Part model, mm, in its own coordinate system. Give positions to 0.01 mm unless a question says otherwise; leave off trailing zeros. Order: outer loops, then holes, each group sorted by start corner. A loop starts at its lowest first (then second) coordinate and runs counter-clockwise, first axis right, second up. Notation, with made-up numbers: M -2,-27 L 45,-27 A22 cw 45,-4 Z; hole C -35,-31 d5. An arc over 180 degrees is marked long. One line per question, with ' | ' between items.
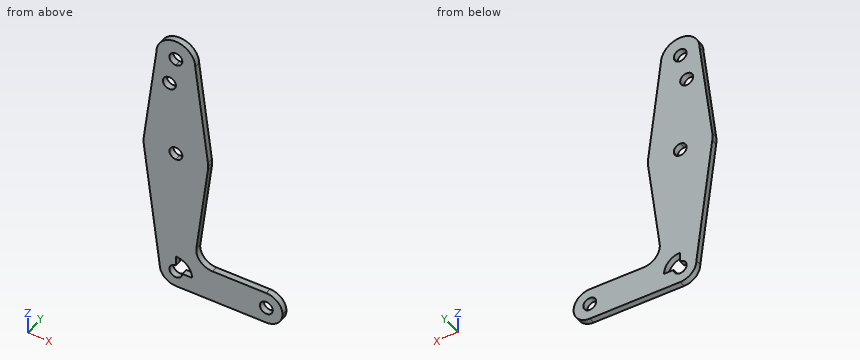
```python
from build123d import *

# Parameters (mm, degrees)
F0_R     = 3.175
F1_DEPTH = 3.048


with BuildPart() as f1:
    # F0 (on Front) → F1 (new body)
    with BuildSketch(Plane.XZ):
        with BuildLine():
            ThreePointArc((3.175, 0), (-2.2450640303, -2.2450640303), (0, 3.175))
            Line((0, 3.175), (0, 7.9375))
            ThreePointArc((0, 7.9375), (-5.6126600757, 5.6126600757), (-7.9375, 0))
            ThreePointArc((-7.9375, 0), (-5.6126600757, -5.6126600757), (0, -7.9375))
            ThreePointArc((0, -7.9375), (5.6126600757, -5.6126600757), (7.9375, 0))
            Line((7.9375, 0), (3.175, 0))
        make_face()
        with BuildLine():
            ThreePointArc((-7.9375, 0), (-5.6126600757, 5.6126600757), (0, 7.9375))
            Line((0, 7.9375), (0, 47.625))
            ThreePointArc((0, 47.625), (-10.4943466753, 51.5884798259), (-15.7484878283, 61.4998109785))
            Line((-15.7484878283, 61.4998109785), (-7.9375, 0))
        make_face()
        with BuildLine():
            Line((0, 47.625), (0, 7.9375))
            ThreePointArc((0, 7.9375), (5.6126600757, 5.6126600757), (7.9375, 0))
            Line((7.9375, 0), (36.5125, 0))
            ThreePointArc((36.5125, 0), (38.8373399243, 5.6126600757), (44.45, 7.9375))
            Line((44.45, 7.9375), (17.969436389, 7.9375))
            ThreePointArc((17.969436389, 7.9375), (12.0041470858, 10.632131185), (10.0825936846, 16.8893946619))
            Line((10.0825936846, 16.8893946619), (15.7484878283, 61.4998109785))
            ThreePointArc((15.7484878283, 61.4998109785), (10.4943466753, 51.5884798259), (0, 47.625))
        make_face()
        with BuildLine():
            Line((36.5125, 0), (7.9375, 0))
            ThreePointArc((7.9375, 0), (5.6126600757, -5.6126600757), (0, -7.9375))
            Line((0, -7.9375), (44.45, -7.9375))
            ThreePointArc((44.45, -7.9375), (38.8373399243, -5.6126600757), (36.5125, 0))
        make_face()
        with BuildLine():
            ThreePointArc((-15.7484878283, 61.4998109785), (-10.4943466753, 51.5884798259), (0, 47.625))
            Line((0, 47.625), (0, 60.325))
            ThreePointArc((0, 60.325), (-3.175, 63.5), (0, 66.675))
            Line((0, 66.675), (0, 79.375))
            ThreePointArc((0, 79.375), (-10.4912828548, 75.4142187767), (-15.7474569047, 65.5082893304))
            ThreePointArc((-15.7474569047, 65.5082893304), (-15.874999475, 63.504082824), (-15.7484878283, 61.4998109785))
        make_face()
        with BuildLine():
            Line((0, 60.325), (0, 47.625))
            ThreePointArc((0, 47.625), (10.4943466753, 51.5884798259), (15.7484878283, 61.4998109785))
            ThreePointArc((15.7484878283, 61.4998109785), (15.8433403876, 62.4979070089), (15.875, 63.5))
            ThreePointArc((15.875, 63.5), (15.8430821396, 64.5061676396), (15.7474569047, 65.5082893304))
            ThreePointArc((15.7474569047, 65.5082893304), (10.4912828548, 75.4142187767), (0, 79.375))
            Line((0, 79.375), (0, 66.675))
            ThreePointArc((0, 66.675), (2.2450640303, 65.7450640303), (3.175, 63.5))
            ThreePointArc((3.175, 63.5), (2.2450640303, 61.2549359697), (0, 60.325))
        make_face()
        with BuildLine():
            ThreePointArc((44.45, 7.9375), (38.8373399243, 5.6126600757), (36.5125, 0))
            ThreePointArc((36.5125, 0), (38.8373399243, -5.6126600757), (44.45, -7.9375))
            ThreePointArc((44.45, -7.9375), (50.0626600757, -5.6126600757), (52.3875, 0))
            ThreePointArc((52.3875, 0), (50.0626600757, 5.6126600757), (44.45, 7.9375))
        make_face()
        with BuildLine():
            ThreePointArc((47.625, 0), (44.45, -3.175), (41.275, 0))
            ThreePointArc((41.275, 0), (44.45, 3.175), (47.625, 0))
        make_face(mode=Mode.SUBTRACT)
        with BuildLine():
            Line((-9.525, 114.3), (-15.7474569047, 65.5082893304))
            ThreePointArc((-15.7474569047, 65.5082893304), (-10.4912828548, 75.4142187767), (0, 79.375))
            Line((0, 79.375), (0, 100.0252))
            Line((0, 100.0252), (0, 104.775))
            ThreePointArc((0, 104.775), (-6.7351920908, 107.5648079092), (-9.525, 114.3))
        make_face()
        with Locations((-3.175, 100.0252)):
            Circle(F0_R, mode=Mode.SUBTRACT)
        with BuildLine():
            Line((0, 100.0252), (0, 79.375))
            ThreePointArc((0, 79.375), (10.4912828548, 75.4142187767), (15.7474569047, 65.5082893304))
            Line((15.7474569047, 65.5082893304), (9.525, 114.3))
            ThreePointArc((9.525, 114.3), (6.7351920908, 107.5648079092), (0, 104.775))
            Line((0, 104.775), (0, 100.0252))
        make_face()
        with BuildLine():
            ThreePointArc((9.525, 114.3), (0, 123.825), (-9.525, 114.3))
            ThreePointArc((-9.525, 114.3), (-6.7351920908, 107.5648079092), (0, 104.775))
            ThreePointArc((0, 104.775), (6.7351920908, 107.5648079092), (9.525, 114.3))
        make_face()
        with BuildLine():
            ThreePointArc((3.175, 114.3), (2.2450640303, 112.0549359697), (0, 111.125))
            ThreePointArc((0, 111.125), (-2.2450640303, 116.5450640303), (3.175, 114.3))
        make_face(mode=Mode.SUBTRACT)
    extrude(amount=F1_DEPTH)


solid = f1.part
```
1. Slice it at B-B on y = -1.1. Give the number of separate pieces and of enclosed holes in the cut face, then the cut area to 3 significant figures.
Worked out:
separate pieces: 1 | enclosed holes: 5 | area: 3,560 mm2
2. Drop flat-ended pins along their axis: pin 1 (1.5 mm diameter, centred on x = 5, y = -1, fed in from +Z); pin 2 (1.5 mm diameter, centred on y = -1.5, z = 6, fed in from +X); pin 3 (1.5 mm diameter, centred on x = -6, y = -2, fed in from -Z). Give the stop position or say it passes through.
Worked out:
pin 1: stops at z = 122.82 | pin 2: stops at x = 50.4 | pin 3: stops at z = -5.95
3. Slice it at D-D on x = 21.5. Give the cut face in (y, z).
Worked out:
outline: M -3.05,-7.94 L 0,-7.94 L 0,7.94 L -3.05,7.94 Z
4. Slice it at A-A on x = -4.5. Give the cut face in (y, z), then the cut area to 3 significant figures.
Worked out:
outline: M -3.05,-6.54 L 0,-6.54 L 0,97.14 L -3.05,97.14 Z; M -3.05,102.91 L 0,102.91 L 0,122.69 L -3.05,122.69 Z | area: 376 mm2
5. Slice it at C-C on z = 89.5. Give the cut face in (x, y).
Worked out:
outline: M -12.69,-3.05 L 12.69,-3.05 L 12.69,0 L -12.69,0 Z
6. Probe L1, parallel to Z at x = 19, y = -0.9; L2, parallel to X at y = -2.5, z = 115; L3, parallel to Z at x = 47, y = -2.55. List the from-to ranges inside material, lowest first. Write a range as from..to.
Worked out:
L1: z = -7.94..7.94 | L2: x = -9.5..-3.1, 3.1..9.5 | L3: z = -7.52..-1.89, 1.89..7.52
